Design review of the part built by this model. Coordinates are the model's own, in mm. Round coordinates to 2 decimals unless told otherwise and drop trailing zeros. Order: outer loops, then holes, each group sorted by start corner. A loop starts at its lowest first (then second) coordinate and runs counter-clockwise, first axis right, second up. Notation, with made-up numbers: (-16.5, 71.5) - (25.5, 71.5) arc R14 ccw to (25.5, 96.5) - close; hole circle Ø8 at (-21, 25). An arc over 180 degrees is marked (long way). Answer as a JSON object with one key per item and string values. Group by question number.
from build123d import *

# Parameters (mm, degrees)
SKETCH1_W           = 457.2
SKETCH1_H           = 381
BOSS_EXTRUDE1_DEPTH = 2
SKETCH119_W         = 50.8
SKETCH119_H         = 101.6
CUT_EXTRUDE1_DEPTH  = 298.577233672
SKETCH120_W         = 101.6
SKETCH120_H         = 127
CUT_EXTRUDE2_DEPTH  = 298.577233672


with BuildPart() as part:
    # Sketch1 → Boss-Extrude1 (new body)
    with BuildSketch(Plane(origin=(0, 0, 0), x_dir=(1, 0, 0), z_dir=(0, 1, 0))):
        Rectangle(SKETCH1_W, SKETCH1_H)
    extrude(amount=BOSS_EXTRUDE1_DEPTH)

    # Sketch119 → Cut-Extrude1 (cut, through all)
    with BuildSketch(Plane(origin=(0, 2, 0), x_dir=(1, 0, 0), z_dir=(0, 1, 0))):
        with Locations((-177.8, 107.95)):
            Rectangle(SKETCH119_W, SKETCH119_H)
        with Locations((177.8, 107.95)):
            Rectangle(SKETCH119_W, SKETCH119_H)
        with Locations((177.8, -107.95)):
            Rectangle(SKETCH119_W, SKETCH119_H)
        with Locations((-177.8, -107.95)):
            Rectangle(SKETCH119_W, SKETCH119_H)
    extrude(amount=-CUT_EXTRUDE1_DEPTH, mode=Mode.SUBTRACT)

    # Sketch120 → Cut-Extrude2 (cut, through all)
    with BuildSketch(Plane(origin=(0, 2, 0), x_dir=(1, 0, 0), z_dir=(0, 1, 0))):
        with Locations((0, -127)):
            Rectangle(SKETCH120_W, SKETCH120_H)
    extrude(amount=-CUT_EXTRUDE2_DEPTH, mode=Mode.SUBTRACT)


solid = part.part
1. Take a section at B-B, the plane y = 0.75. Give the boundary of the cut face in (x, z), then the cut area to 3 significant figures.
2. Clearance check with a flat-ended pin moving along its axis: P1, Ø5, axis at x = -27, z = -50, coming from the -Y side. State where the tip first meets the part, or that it passes through.
3. Take a section at D-D, the plane z = -109. Give the boundary of the cut face in (x, y), then the cut area to 3 significant figures.
4. To check wall thickness, follow line 1 (X direction, y = 1.75, z = -128.5); line 2 (X direction, y = 1.75, z = 118.5); line 3 (Z direction, x = 169, y = 1.85). State the ranges of each line that lie inside material, in increasing order. Write a range as from..to.
5. Take a section at A-A, the plane z = 94.5. Give the boundary of the cut face in (x, y), then the cut area to 3 significant figures.
6. Take a section at C-C, the plane x = -162.5. Give the boundary of the cut face in (y, z), then the cut area to 3 significant figures.
Response values:
{
 "1": {"outline": "(-228.6, -190.5) - (228.6, -190.5) - (228.6, 190.5) - (50.8, 190.5) - (50.8, 63.5) - (-50.8, 63.5) - (-50.8, 190.5) - (-228.6, 190.5) - close; hole (-203.2, -158.75) - (-152.4, -158.75) - (-152.4, -57.15) - (-203.2, -57.15) - close; hole (-203.2, 57.15) - (-152.4, 57.15) - (-152.4, 158.75) - (-203.2, 158.75) - close; hole (152.4, -158.75) - (203.2, -158.75) - (203.2, -57.15) - (152.4, -57.15) - close; hole (152.4, 57.15) - (203.2, 57.15) - (203.2, 158.75) - (152.4, 158.75) - close", "area": "141,000 mm2"},
 "2": {"P1": "y = 0"},
 "3": {"outline": "(-228.6, 0) - (-203.2, 0) - (-203.2, 2) - (-228.6, 2) - close; (-152.4, 0) - (152.4, 0) - (152.4, 2) - (-152.4, 2) - close; (203.2, 0) - (228.6, 0) - (228.6, 2) - (203.2, 2) - close", "area": "711 mm2"},
 "4": {"line 1": "-228.6..-203.2, -152.4..152.4, 203.2..228.6", "line 2": "-228.6..-203.2, -152.4..-50.8, 50.8..152.4, 203.2..228.6", "line 3": "-190.5..-158.75, -57.15..57.15, 158.75..190.5"},
 "5": {"outline": "(-228.6, 0) - (-203.2, 0) - (-203.2, 2) - (-228.6, 2) - close; (-152.4, 0) - (-50.8, 0) - (-50.8, 2) - (-152.4, 2) - close; (50.8, 0) - (152.4, 0) - (152.4, 2) - (50.8, 2) - close; (203.2, 0) - (228.6, 0) - (228.6, 2) - (203.2, 2) - close", "area": "508 mm2"},
 "6": {"outline": "(0, -190.5) - (2, -190.5) - (2, -158.75) - (0, -158.75) - close; (0, -57.15) - (2, -57.15) - (2, 57.15) - (0, 57.15) - close; (0, 158.75) - (2, 158.75) - (2, 190.5) - (0, 190.5) - close", "area": "356 mm2"}
}
